from build123d import *

# Parameters (mm, degrees)
BOSS_EXTRUDE2_DEPTH      = 11.25
BOSS_EXTRUDE2_DEPTH_BACK = 11.25
SKETCH4_R                = 3.175
BOSS_EXTRUDE3_DEPTH      = 7.0000114


with BuildPart() as part:
    # Sketch3 → Boss-Extrude2 (new body, two sides)
    with BuildSketch(Plane.XY) as boss_extrude2_sk:
        Polygon((-5.55625, -3.207902433), (0, -6.415804866), (5.55625, -3.207902433), (5.55625, 3.207902433), (0, 6.415804866), (-5.55625, 3.207902433), align=None)
    extrude(amount=BOSS_EXTRUDE2_DEPTH)
    extrude(boss_extrude2_sk.sketch, amount=-BOSS_EXTRUDE2_DEPTH_BACK)

    # Sketch4 → Boss-Extrude3 (add)
    with BuildSketch(Plane.XY.offset(-11.25)):
        Circle(SKETCH4_R)
    extrude(amount=-BOSS_EXTRUDE3_DEPTH)


solid = part.part
Input: part model. Units: mm. Frame: model coordinates. A direction names the side the tool comes from. Give positions to 0.01 mm unless a question says otherwise; leave off trailing zeros. Order: outer loops, then holes, each group sorted by start corner. A loop starts at its lowest first (then second) coordinate and runs counter-clockwise, first axis right, second up. Notation, with made-up numbers: (-25, 49) -> (16, 49) arc R22 cw to (16, 87) -> close; hole circle Ø5 at (75, 65.5). An arc over 180 degrees is marked (long way). Use one line per item in the form item = value.
1) Section A-A, the plane y = 0. Return loops of the section in (x, z) (3 decimals).
Response values:
outline = (-5.556, -11.25) -> (-3.175, -11.25) -> (-3.175, -18.25) -> (3.175, -18.25) -> (3.175, -11.25) -> (5.556, -11.25) -> (5.556, 11.25) -> (-5.556, 11.25) -> close
2) Reachability of faces 1 (the cylindrical face through (-0.69, -3.1, -14.7)), 2 (the flat face through (-2.739, 4.834, 0.158)) from +Z, -Z, +X, -X, +Y, -Y: full face, straight path, thin tool, end or side. Return the list, or none.
Response values:
face_1 = -Z
face_2 = +Z, -Z, -X, +Y
3) Line query: probe 1 along Z at (x, y) = (2.25, -3.75); probe 2 along Y at (x, z) = (-1.75, -13.25); probe 3 along Y at (x, z) = (-2, -13.25). Output: solid intervals per line, ascending.
Response values:
probe_1 = -11.25 to 11.25
probe_2 = -2.65 to 2.65
probe_3 = -2.47 to 2.47
4) Section B-B, the plane z = 2.5. Return loops of the section in (x, y), and give its area (3 significant figures).
Response values:
outline = (-5.56, -3.21) -> (0, -6.42) -> (5.56, -3.21) -> (5.56, 3.21) -> (0, 6.42) -> (-5.56, 3.21) -> close
area = 107 mm^2
5) First-contact query: pin 1 Ø5 at (y, z) = (2.5, -14) entering from +X (3 decimals); pin 2 Ø4 at (x, z) = (4.5, 6.5) entering from +Y; pin 3 Ø1.5 at (x, z) = (3.5, -14) entering from +Y. Flat tips, straight axial feed; report the tip coordinate or a pass-through.
Response values:
pin_1 = 3.175
pin_2 = 4.97
pin_3 = 1.59
6) Section C-C, the plane y = -2.5. Return loops of the section in (x, z).
Response values:
outline = (-5.56, -11.25) -> (-1.96, -11.25) -> (-1.96, -18.25) -> (1.96, -18.25) -> (1.96, -11.25) -> (5.56, -11.25) -> (5.56, 11.25) -> (-5.56, 11.25) -> close
7) Section D-D, the plane z = -15. Return loops of the section in (x, y) (3 decimals), and give its area (3 significant figures).
Response values:
outline = circle Ø6.35 at (0, 0)
area = 31.7 mm^2
